Could you check a few things on this model? Use its own coordinates, in mm. Face numbers are marked on the shaded views. Round coordinates to 2 decimals unless told otherwise and drop trailing zeros. Loops run counter-clockwise (first coordinate to the right, second up) from the corner with the lowest first, then second, coordinate; pieces in that order, holes last. Notation, with made-up numbers: (-28.75, -35.75) -> (2.25, -35.75) arc R26 cw to (2.25, -17.75) -> close; hole circle Ø6 at (63.25, 12.25). An arc over 180 degrees is marked (long way). One line per item, written item: value.
from build123d import *

# Parameters (mm, degrees)
SKETCH1_R           = 3.25
SKETCH1_R_2         = 2.5
BOSS_EXTRUDE1_DEPTH = 3
BOSS_EXTRUDE2_START = -9.65
SKETCH2_W           = 11
SKETCH2_H           = 16
BOSS_EXTRUDE2_DEPTH = 2


with BuildPart() as part:
    # Sketch1 → Boss-Extrude1 (new body)
    with BuildSketch(Plane(origin=(0, 0, 0), x_dir=(0, 0, -1), z_dir=(1, 0, 0))):
        with BuildLine():
            Line((0, 6.35), (38.1, 6.35))
            ThreePointArc((38.1, 6.35), (44.45, 0), (38.1, -6.35))
            Line((38.1, -6.35), (32.5, -6.35))
            ThreePointArc((32.5, -6.35), (31.792893219, -6.642893219), (31.5, -7.35))
            Line((31.5, -7.35), (31.5, -9.65))
            Line((31.5, -9.65), (15.5, -9.65))
            Line((15.5, -9.65), (15.5, -7.35))
            ThreePointArc((15.5, -7.35), (15.207106781, -6.642893219), (14.5, -6.35))
            Line((14.5, -6.35), (0, -6.35))
            ThreePointArc((0, -6.35), (-6.35, 0), (0, 6.35))
        make_face()
        Circle(SKETCH1_R, mode=Mode.SUBTRACT)
        with Locations((38.1, 0)):
            Circle(SKETCH1_R_2, mode=Mode.SUBTRACT)
    extrude(amount=BOSS_EXTRUDE1_DEPTH)

    # Sketch2 → Boss-Extrude2 (add)
    with BuildSketch(Plane(origin=(0, 0, 0), x_dir=(1, 0, 0), z_dir=(0, 1, 0)).offset(BOSS_EXTRUDE2_START)):
        with Locations((8.5, 23.5)):
            Rectangle(SKETCH2_W, SKETCH2_H)
    extrude(amount=BOSS_EXTRUDE2_DEPTH)

    # Mirror2: part across plane


with BuildPart() as part_1:
    add(part.part)
    add(part.part.mirror(Plane(origin=(14, 0, 0), x_dir=(0, 0, 1), z_dir=(1, 0, 0))))


solid = part_1.part
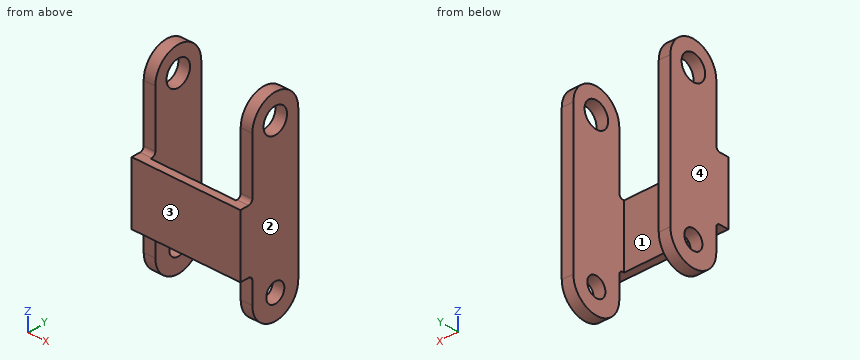
(1) If we section it at C-C, the plane z = 2.5: Please give me the cut outline in (x, y).
Recorded:
outline: (0, -5.84) -> (3, -5.84) -> (3, -2.08) -> (0, -2.08) -> close; (0, 2.08) -> (3, 2.08) -> (3, 5.84) -> (0, 5.84) -> close; (25, -5.84) -> (28, -5.84) -> (28, -2.08) -> (25, -2.08) -> close; (25, 2.08) -> (28, 2.08) -> (28, 5.84) -> (25, 5.84) -> close
(2) If I drill on L1, parallel to X at y = -4, z = -1.5; L2, parallel to Y at x = 19.5, z = -18.5; L3, parallel to Y at x = 1.2, z = -38.1, over which ranges is the centre line in solid material (lowest first)?
Recorded:
L1: 0 to 3, 25 to 28
L2: -9.65 to -7.65
L3: -6.35 to -2.5, 2.5 to 6.35
(3) I'm going to push flat-ended pins straight in: pin 1 Ø6 at (y, z) = (0, 0) entering from +X; pin 2 Ø13 at (x, z) = (12, -22.5) entering from +Y; pin 3 Ø2.5 at (x, z) = (1, -10) entering from -Y; pin 4 Ø1.5 at (x, y) = (24.5, 2) entering from -Z. Where does each tip first touch, or does it pass through?
Recorded:
pin 1: through
pin 2: y = -7.65
pin 3: y = -6.35
pin 4: z = -44.28
(4) If we section it at B-B, the plane y = -5.75: Please give me the cut outline in (x, z).
Recorded:
outline: (0, -40.79) -> (3, -40.79) -> (3, 2.69) -> (0, 2.69) -> close; (25, -40.79) -> (28, -40.79) -> (28, 2.69) -> (25, 2.69) -> close
(5) If we section it at D-D, the plane z = -20: Please give me the cut outline in (x, y), then the cut area to 3 significant figures.
Recorded:
outline: (0, -9.65) -> (28, -9.65) -> (28, 6.35) -> (25, 6.35) -> (25, -7.65) -> (3, -7.65) -> (3, 6.35) -> (0, 6.35) -> close
area: 140 mm²
(6) Thinking about a two-plate mould opening in X: for the marked faces 1, 2, 3 and 4, which applies, released by +X, released by -X, zero draft, split by the parting line, or undercut?
Recorded:
face 1: undercut
face 2: released by +X
face 3: zero draft
face 4: released by -X
(7) If we section it at A-A, the plane y = 0: Please give me the cut outline in (x, z).
Recorded:
outline: (0, -44.45) -> (3, -44.45) -> (3, -40.6) -> (0, -40.6) -> close; (0, -35.6) -> (3, -35.6) -> (3, -3.25) -> (0, -3.25) -> close; (0, 3.25) -> (3, 3.25) -> (3, 6.35) -> (0, 6.35) -> close; (25, -44.45) -> (28, -44.45) -> (28, -40.6) -> (25, -40.6) -> close; (25, -35.6) -> (28, -35.6) -> (28, -3.25) -> (25, -3.25) -> close; (25, 3.25) -> (28, 3.25) -> (28, 6.35) -> (25, 6.35) -> close
